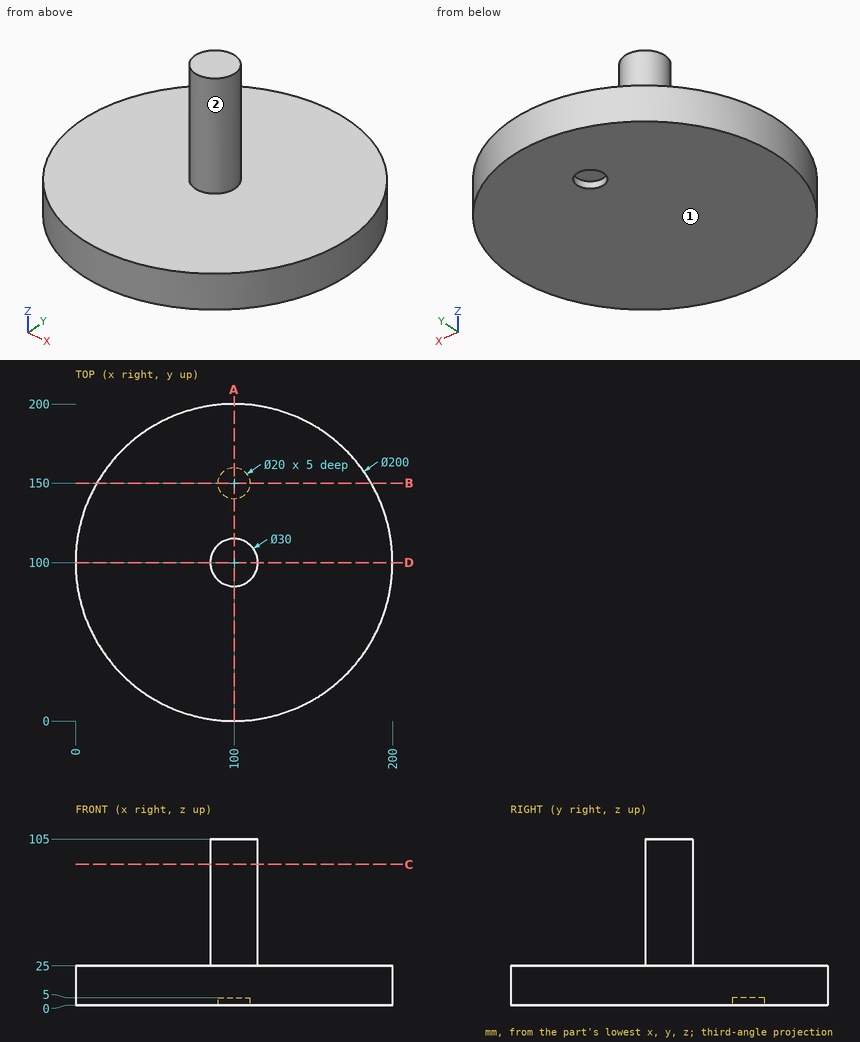
Input: dimensioned drawing with shaded views. Units: mm. Origin: part minimum x, y, z. A direction names the side the tool comes from. Give positions to 0.01 mm unless a question says otherwise; leave off trailing zeros. Write each loop counter-clockwise with the first axis right and the second up, starting at its lowest first coordinate (ties: lowest second). Pieces come first, ordered by that corner, then holes. Notation, with made-up numbers: M 14,63 L 44,63 A20 cw 44,98 Z; hole C 71,-25.5 d8. An arc over 180 degrees is marked long. Return JSON: item names as keys, results as strings. Group by question number.
1) Material intervals for line 1 along Y through (x, z) = (100, 1.5); line 2 along Z through (x, y) = (152.5, 111); line 3 along Z through (x, y) = (95, 143), sorted ascending. Write a range as [from, to].
2) Cut plane A-A, the plane x = 100. Output: boundary loops of the cut face in (y, z).
3) Cut plane B-B, the plane y = 150. Output: boundary loops of the cut face in (x, z).
4) Cut plane C-C, the plane z = 89. Output: boundary loops of the cut face in (x, y).
5) Cut plane D-D, the plane y = 100. Output: boundary loops of the cut face in (x, z), plus the area to 3 significant figures.
6) Set-up query: the marked faces 1 and 2. Return all of +Z, -Z, +X, -X, +Y, -Y with unobstructed straight access to the full face (end or side cutting, diameter ignored); none if empty.
7) Pin query (flat end, axial travel): P1, Ø5, axis at x = 116.5, y = 127, coming from the +Z side; P2, Ø12, axis at x = 97, z = 76, coming from the -Y side; P3, Ø3, axis at x = 48.5, z = 23, coming from the -Y side. Return the tip coordinate at first contact, or that it passes through.
Recorded:
{
 "1": {"line 1": "y = [0, 140], [160, 200]", "line 2": "z = [0, 25]", "line 3": "z = [5, 25]"},
 "2": {"outline": "M 0,0 L 140,0 L 140,5 L 160,5 L 160,0 L 200,0 L 200,25 L 115,25 L 115,105 L 85,105 L 85,25 L 0,25 Z"},
 "3": {"outline": "M 13.4,0 L 90,0 L 90,5 L 110,5 L 110,0 L 186.6,0 L 186.6,25 L 13.4,25 Z"},
 "4": {"outline": "C 100,100 d30"},
 "5": {"outline": "M 0,0 L 200,0 L 200,25 L 115,25 L 115,105 L 85,105 L 85,25 L 0,25 Z", "area": "7,400 mm²"},
 "6": {"face 1": "-Z, +X, -X, +Y, -Y", "face 2": "+Z"},
 "7": {"P1": "stops at z = 25", "P2": "stops at y = 85", "P3": "stops at y = 13.4"}
}
